Input: part model. Units: mm. Frame: model coordinates. Coordinates: 2 decimals unless noted, no trailing zeros. Loops run counter-clockwise (first coordinate to the right, second up) from the corner with the lowest first, then second, coordinate; pieces in that order, holes last. Notation, with made-up numbers: M -33.75,34 L 24.25,34 A7 cw 24.25,45 Z; hole C 24,83.25 d6. An arc over 180 degrees is marked long. Use a Markdown table: item, result. Add a question column.
1. Line query: L1, parallel to X at y = 7, z = 0; L2, parallel to X at y = 66, z = 30; L3, parallel to Z at x = 25.5, y = 29. Output: solid intervals per line, ascending. Write a range as [from, to].
2. Section C-C on y = 8. Output: boundary loops of the cut face in (x, z).
3. Pin query (flat end, axial travel): pin 1 (4 mm diameter, centred on x = 22.9, z = 0, fed in from +Y); pin 2 (5.5 mm diameter, centred on x = 5.9, y = 54.31, fed in from -Z). Return the tip coordinate at first contact, or that it passes through.
4. Section A-A on z = 0. Output: boundary loops of the cut face in (x, y).
5. Section B-B on x = 10. Output: boundary loops of the cut face in (y, z), then the cut area to 3 significant figures.
6. Section D-D on y = 30. Output: boundary loops of the cut face in (x, z).
```python
from build123d import *

# Parameters (mm, degrees)
SKETCH5_W           = 34
SKETCH5_H           = 34
BOSS_EXTRUDE1_DEPTH = 13.19
SKETCH6_W           = 34
SKETCH6_H           = 87.79
BOSS_EXTRUDE2_DEPTH = 23.83
SKETCH7_R           = 3
CUT_EXTRUDE1_DEPTH  = 21.83
SKETCH8_R           = 1.72
CUT_EXTRUDE2_DEPTH  = 31.83
SKETCH9_R           = 1.72
CUT_EXTRUDE3_DEPTH  = 31.83
RIB18_REACH         = 103.535
SKETCH20_WALL_W     = 212.140430626
SKETCH20_WALL_H     = 2
RIB19_REACH         = 103.535
SKETCH21_WALL_W     = 212.140430626
SKETCH21_WALL_H     = 2


with BuildPart() as part:
    # Sketch5 → Boss-Extrude1 (new body)
    with BuildSketch(Plane(origin=(0, 0, 0), x_dir=(1, 0, 0), z_dir=(0, 1, 0))):
        with Locations((14.397550388, 1.103341085)):
            Rectangle(SKETCH5_W, SKETCH5_H)
    extrude(amount=BOSS_EXTRUDE1_DEPTH)

    # Sketch6 → Boss-Extrude2 (add)
    with BuildSketch(Plane.XY.offset(15.896658915)):
        with Locations((14.397550388, 43.895)):
            Rectangle(SKETCH6_W, SKETCH6_H)
    extrude(amount=BOSS_EXTRUDE2_DEPTH)

    # Sketch7 → Cut-Extrude1 (cut)
    with BuildSketch(Plane(origin=(0, 13.19, 0), x_dir=(1, 0, 0), z_dir=(0, 1, 0))):
        with Locations(Location((14.397550388, 0, 0), (0, 0, 270))):
            Circle(SKETCH7_R)
    extrude(amount=-CUT_EXTRUDE1_DEPTH, mode=Mode.SUBTRACT)

    # Sketch8 → Cut-Extrude2 (cut)
    with BuildSketch(Plane.XY.offset(39.726658915)):
        with Locations((5.897550388, 66.793195428)):
            Circle(SKETCH8_R)
        with Locations((22.897550388, 66.793195428)):
            Circle(SKETCH8_R)
        with Locations((5.897550388, 54.310639336)):
            Circle(SKETCH8_R)
        with Locations((22.897550388, 54.310639336)):
            Circle(SKETCH8_R)
    extrude(amount=-CUT_EXTRUDE2_DEPTH, mode=Mode.SUBTRACT)

    # Sketch9 → Cut-Extrude3 (cut)
    with BuildSketch(Plane(origin=(0, 13.19, 0), x_dir=(1, 0, 0), z_dir=(0, 1, 0))):
        with Locations(Location((22.897550388, 0, 0), (0, 0, 270))):
            Circle(SKETCH9_R)
        with Locations(Location((14.369066497, 9.603341085, 0), (0, 0, 270))):
            Circle(SKETCH9_R)
        with Locations(Location((14.369066497, -7.396658915, 0), (0, 0, 270))):
            Circle(SKETCH9_R)
        with Locations(Location((5.897550388, 0, 0), (0, 0, 270))):
            Circle(SKETCH9_R)
    extrude(amount=-CUT_EXTRUDE3_DEPTH, mode=Mode.SUBTRACT)

    # Sketch20 wall → Rib18 (add, up to next)
    with BuildSketch(Plane(origin=(-0.602449612, 15.69, 13.396658915), x_dir=(0, 0.707106781187, 0.707106781187), z_dir=(0, 0.707106781187, -0.707106781187)), mode=Mode.PRIVATE) as rib18_sk1:
        with Locations((0, -1)):
            Rectangle(SKETCH20_WALL_W, SKETCH20_WALL_H)
    rib18_tool1 = extrude(rib18_sk1.sketch, amount=-RIB18_REACH, mode=Mode.PRIVATE) - part.part
    add(rib18_tool1.solids().sort_by_distance((-0.602449612, 15.69, 13.396658915))[0])

    # Sketch21 wall → Rib19 (add, up to next)
    with BuildSketch(Plane(origin=(29.397550388, 15.69, 13.396658915), x_dir=(0, -0.707106781187, -0.707106781187), z_dir=(0, 0.707106781187, -0.707106781187)), mode=Mode.PRIVATE) as rib19_sk1:
        with Locations((0, -1)):
            Rectangle(SKETCH21_WALL_W, SKETCH21_WALL_H)
    rib19_tool1 = extrude(rib19_sk1.sketch, amount=-RIB19_REACH, mode=Mode.PRIVATE) - part.part
    add(rib19_tool1.solids().sort_by_distance((29.397550388, 15.69, 13.396658915))[0])


solid = part.part
```
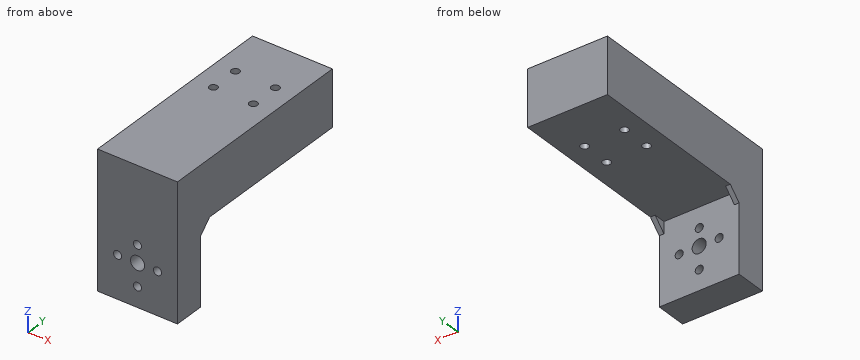
Answers below:
| question | item | result |
|---|---|---|
| 1 | L1 | x = [-2.6, 4.18], [7.62, 11.4], [17.4, 21.18], [24.62, 31.4] |
| 1 | L2 | x = [-2.6, 4.37], [7.42, 21.37], [24.42, 31.4] |
| 1 | L3 | z = [15.9, 39.73] |
| 2 | outline | M -2.6,-18.1 L 31.4,-18.1 L 31.4,39.73 L -2.6,39.73 Z; hole C 5.9,0 d3.44; hole C 14.4,0 d6; hole C 14.37,-9.6 d3.44; hole C 14.37,7.4 d3.44; hole C 22.9,0 d3.44 |
| 3 | pin 1 | stops at y = 13.19 |
| 3 | pin 2 | stops at z = 15.9 |
| 4 | outline | M -2.6,0 L 4.18,0 L 4.18,13.19 L -2.6,13.19 Z; M 7.62,0 L 11.4,0 L 11.4,13.19 L 7.62,13.19 Z; M 17.4,0 L 21.18,0 L 21.18,13.19 L 17.4,13.19 Z; M 24.62,0 L 31.4,0 L 31.4,13.19 L 24.62,13.19 Z |
| 5 | outline | M 0,-18.1 L 13.19,-18.1 L 13.19,15.9 L 87.79,15.9 L 87.79,39.73 L 0,39.73 Z |
| 5 | area | 2,540 mm² |
| 6 | outline | M -2.6,15.9 L 31.4,15.9 L 31.4,39.73 L -2.6,39.73 Z |
